```python
from build123d import *

# Parameters (mm, degrees)
BOSS_EXTRUDE1_DEPTH = 406.4
SKETCH3_W           = 193.04
SKETCH3_H           = 152.4
BOSS_EXTRUDE2_DEPTH = 152.4
SKETCH4_W           = 30.48
SKETCH4_H           = 254
BOSS_EXTRUDE3_DEPTH = 144.78
SKETCH5_R           = 38.1
CUT_EXTRUDE1_DEPTH  = 193.04
FILLET1_R           = 76.2
CHAMFER2_SIZE       = 144.78
CHAMFER2_SIZE2      = 296.926


with BuildPart() as part:
    # Sketch2 → Boss-Extrude1 (new body)
    with BuildSketch(Plane.XY):
        Polygon((-96.52, 5.08), (-127, 5.08), (-127, -25.4), (-66.04, -25.4), (-66.04, 0), (66.04, 0), (66.04, -25.4), (127, -25.4), (127, 5.08), (96.52, 5.08), (96.52, 35.56), (-96.52, 35.56), align=None)
    extrude(amount=BOSS_EXTRUDE1_DEPTH)

    # Sketch3 → Boss-Extrude2 (add)
    with BuildSketch(Plane(origin=(0, 35.56, 0), x_dir=(1, 0, 0), z_dir=(0, 1, 0))):
        with Locations((0, -76.2)):
            Rectangle(SKETCH3_W, SKETCH3_H)
    extrude(amount=BOSS_EXTRUDE2_DEPTH)

    # Sketch4 → Boss-Extrude3 (add)
    with BuildSketch(Plane(origin=(0, 35.56, 0), x_dir=(1, 0, 0), z_dir=(0, 1, 0))):
        with Locations((0, -279.4)):
            Rectangle(SKETCH4_W, SKETCH4_H)
    extrude(amount=BOSS_EXTRUDE3_DEPTH)

    # Sketch5 → Cut-Extrude1 (cut)
    with BuildSketch(Plane(origin=(96.52, 0, 0), x_dir=(0, 0, -1), z_dir=(1, 0, 0))):
        with Locations((-76.2, 111.76)):
            Circle(SKETCH5_R)
    extrude(amount=-CUT_EXTRUDE1_DEPTH, mode=Mode.SUBTRACT)

    # Fillet1
    # the kernel refuses this fillet: 76.2 mm, written as the material it takes off along each edge
    with BuildSketch(Plane(origin=(287.02, 187.96, 152.4), x_dir=(0, -1, 0), z_dir=(-1, 0, 0))) as fillet1_piece_1_section:
        with BuildLine():
            CenterArc((FILLET1_R, -FILLET1_R), FILLET1_R, 90, 90)
            Line((0, -FILLET1_R), (0, 0))
            Line((0, 0), (FILLET1_R, 0))
        make_face()
    fillet1_piece_1 = extrude(amount=574.04, mode=Mode.PRIVATE)
    fillet1_piece_1 = split(fillet1_piece_1, bisect_by=Plane(origin=(15.24, 162.276069746, 141.915616322), z_dir=(1, 0, 0)), keep=Keep.TOP, mode=Mode.PRIVATE)
    fillet1_piece_1 = split(fillet1_piece_1, bisect_by=Plane(origin=(151.13, 180.34, 141.915616322), z_dir=(0, -1, 0)), keep=Keep.TOP, mode=Mode.PRIVATE)
    add(fillet1_piece_1, mode=Mode.SUBTRACT)
    with BuildSketch(Plane(origin=(287.02, 187.96, 152.4), x_dir=(0, -1, 0), z_dir=(-1, 0, 0))) as fillet1_piece_2_section:
        with BuildLine():
            CenterArc((FILLET1_R, -FILLET1_R), FILLET1_R, 90, 90)
            Line((0, -FILLET1_R), (0, 0))
            Line((0, 0), (FILLET1_R, 0))
        make_face()
    fillet1_piece_2 = extrude(amount=574.04, mode=Mode.PRIVATE)
    fillet1_piece_2 = split(fillet1_piece_2, bisect_by=Plane(origin=(15.24, 185.388736326, 123.368401859), z_dir=(1, 0, 0)), keep=Keep.TOP, mode=Mode.PRIVATE)
    fillet1_piece_2 = split(fillet1_piece_2, bisect_by=Plane(origin=(151.13, 180.34, 123.368401859), z_dir=(0, 1, 0)), keep=Keep.TOP, mode=Mode.PRIVATE)
    add(fillet1_piece_2, mode=Mode.SUBTRACT)
    with BuildSketch(Plane(origin=(287.02, 187.96, 152.4), x_dir=(0, -1, 0), z_dir=(-1, 0, 0))) as fillet1_piece_3_section:
        with BuildLine():
            CenterArc((FILLET1_R, -FILLET1_R), FILLET1_R, 90, 90)
            Line((0, -FILLET1_R), (0, 0))
            Line((0, 0), (FILLET1_R, 0))
        make_face()
    fillet1_piece_3 = extrude(amount=574.04, mode=Mode.PRIVATE)
    fillet1_piece_3 = split(fillet1_piece_3, bisect_by=Plane(origin=(15.24, 185.388736326, 123.368401859), z_dir=(-1, 0, 0)), keep=Keep.TOP, mode=Mode.PRIVATE)
    fillet1_piece_3 = split(fillet1_piece_3, bisect_by=Plane(origin=(0, 180.34, 123.368401859), z_dir=(0, 1, 0)), keep=Keep.TOP, mode=Mode.PRIVATE)
    fillet1_piece_3 = split(fillet1_piece_3, bisect_by=Plane(origin=(-15.24, 185.388736326, 123.368401859), z_dir=(1, 0, 0)), keep=Keep.TOP, mode=Mode.PRIVATE)
    add(fillet1_piece_3, mode=Mode.SUBTRACT)
    with BuildSketch(Plane(origin=(287.02, 187.96, 152.4), x_dir=(0, -1, 0), z_dir=(-1, 0, 0))) as fillet1_piece_4_section:
        with BuildLine():
            CenterArc((FILLET1_R, -FILLET1_R), FILLET1_R, 90, 90)
            Line((0, -FILLET1_R), (0, 0))
            Line((0, 0), (FILLET1_R, 0))
        make_face()
    fillet1_piece_4 = extrude(amount=574.04, mode=Mode.PRIVATE)
    fillet1_piece_4 = split(fillet1_piece_4, bisect_by=Plane(origin=(-151.13, 180.34, 141.915616322), z_dir=(0, -1, 0)), keep=Keep.TOP, mode=Mode.PRIVATE)
    fillet1_piece_4 = split(fillet1_piece_4, bisect_by=Plane(origin=(-15.24, 162.276069746, 141.915616322), z_dir=(-1, 0, 0)), keep=Keep.TOP, mode=Mode.PRIVATE)
    add(fillet1_piece_4, mode=Mode.SUBTRACT)
    with BuildSketch(Plane(origin=(287.02, 187.96, 152.4), x_dir=(0, -1, 0), z_dir=(-1, 0, 0))) as fillet1_piece_5_section:
        with BuildLine():
            CenterArc((FILLET1_R, -FILLET1_R), FILLET1_R, 90, 90)
            Line((0, -FILLET1_R), (0, 0))
            Line((0, 0), (FILLET1_R, 0))
        make_face()
    fillet1_piece_5 = extrude(amount=574.04, mode=Mode.PRIVATE)
    fillet1_piece_5 = split(fillet1_piece_5, bisect_by=Plane(origin=(-151.13, 180.34, 123.368401859), z_dir=(0, 1, 0)), keep=Keep.TOP, mode=Mode.PRIVATE)
    fillet1_piece_5 = split(fillet1_piece_5, bisect_by=Plane(origin=(-15.24, 185.388736326, 123.368401859), z_dir=(-1, 0, 0)), keep=Keep.TOP, mode=Mode.PRIVATE)
    add(fillet1_piece_5, mode=Mode.SUBTRACT)
    with BuildSketch(Plane(origin=(-287.02, 187.96, 0), x_dir=(0, -1, 0), z_dir=(1, 0, 0))) as fillet1_piece_6:
        with BuildLine():
            CenterArc((FILLET1_R, -FILLET1_R), FILLET1_R, 90, 90)
            Line((0, -FILLET1_R), (0, 0))
            Line((0, 0), (FILLET1_R, 0))
        make_face()
    extrude(amount=574.04, mode=Mode.SUBTRACT)

    # Chamfer2
    chamfer2_edges = [part.edges().sort_by_distance(p)[0] for p in [
        (0, 180.34, 406.4),
    ]]
    chamfer2_side = [part.faces().sort_by_distance(p)[0] for p in [
        (0, 38.129015817, 406.4),
    ]]
    chamfer(chamfer2_edges, length=CHAMFER2_SIZE, length2=CHAMFER2_SIZE2, reference=chamfer2_side[0])


solid = part.part
```
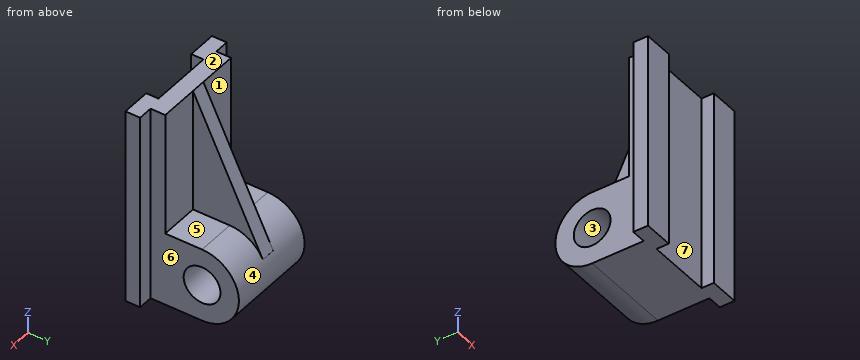
The model under review builds one solid part; all positions refer to its coordinate system, in mm. Face numbers are marked on the shaded views. A direction names the side the tool comes from. Round coordinates to 2 decimals unless told otherwise and drop trailing zeros. Write each loop counter-clockwise with the first axis right and the second up, starting at its lowest first coordinate (ties: lowest second). Pieces come first, ordered by that corner, then holes. Notation, with made-up numbers: (53, -6.5) - (105, -6.5) arc R8 cw to (105, 4.5) - close; hole circle Ø4 at (72, -20.75). An arc over 180 degrees is marked (long way). Answer as CSV lines item,"result". Start each with the question number.
(1) We need section C-C on y = 99. State the section outline as (x, z) points.
(2) We need section B-B on x = -90. State the section outline as (y, z) points, plus the area to 3 significant figures.
(3) We need section D-D on x = -1. State the section outline as (y, z) points.
(4) For pin 1 Ø6 at (x, y) = (84, 126) entering from -Z; pin 2 Ø3 at (y, z) = (166, 87.5) entering from +X; pin 3 Ø24.5 at (x, z) = (110, 151) entering from +Y; pin 4 Ø2 at (x, y) = (98.5, 59.5) entering from +Z, all flat-tipped, find the tip position at first contact; note any pin that passes through.
(5) Draft analysis for pull direction Z (two halves, no side actions). For the marked faces 1, 2 and 3, state which applies: pulls with the +Z half, pulls with the -Z half, needs draft (parallel to the pull), parting line crosses it, or undercut.
(6) We need section A-A on z = 76.2. State the section outline as (x, y) points.
(7) For the marked faces 4, 5, 6 and 7, list the 3-axis set-ups (+Z, -Z, +X, -X, +Y, -Y) from which the entire face can be reached by the end or side of a thin tool; tool diameter is ignored.
(8) To check wall thickness, follow line 1 (Y direction, x = -52, z = 76); line 2 (X direction, y = 57, z = 170.5); line 3 (Y direction, x = 92.5, z = 239). State the ranges of each line that lie inside material, in increasing order.
Worked answers:
1,outline,"(-96.52, 0) - (96.52, 0) - (96.52, 40.3) - (-96.52, 40.3) - close; (-96.52, 112.1) - (96.52, 112.1) - (96.52, 152.4) - (15.24, 152.4) - (15.24, 276.29) - (-15.24, 276.29) - (-15.24, 152.4) - (-96.52, 152.4) - close"
2,outline,"(-25.4, 0) - (111.76, 0) arc R76.2 ccw to (111.76, 152.4) - (35.56, 152.4) - (35.56, 406.4) - (-25.4, 406.4) - close; hole circle Ø76.2 at (111.76, 76.2)"
2,area,"40,900 mm²"
3,outline,"(0, 0) - (111.76, 0) arc R76.2 ccw to (180.34, 109.41) - (180.34, 109.47) - (35.56, 406.4) - (0, 406.4) - close; hole circle Ø76.2 at (111.76, 76.2)"
4,pin 1,"z = 0.83"
4,pin 2,"x = 96.52"
4,pin 3,"y = 5.08"
4,pin 4,"through"
5,face 1,"needs draft"
5,face 2,"pulls with the +Z half"
5,face 3,"undercut"
6,outline,"(-127, -25.4) - (-66.04, -25.4) - (-66.04, 0) - (66.04, 0) - (66.04, -25.4) - (127, -25.4) - (127, 5.08) - (96.52, 5.08) - (96.52, 73.66) - (-96.52, 73.66) - (-96.52, 5.08) - (-127, 5.08) - close; (-96.52, 149.86) - (96.52, 149.86) - (96.52, 187.96) - (-96.52, 187.96) - close"
7,face 4,"+Y"
7,face 5,"+Z, +X, +Y"
7,face 6,"+Z, -Z, +X, +Y"
7,face 7,"+Z, -Z, -Y"
8,line 1,"0 to 73.66, 149.86 to 187.96"
8,line 2,"-15.24 to 15.24"
8,line 3,"-25.4 to 35.56"
